```python
from build123d import *

# Parameters (mm, degrees)
EXTRUSION1_DEPTH = 240
ESQUISSE2_R      = 1.5
EXTRUSION2_DEPTH = 242.541404318
ESQUISSE3_W      = 1.5
ESQUISSE3_H      = 20
EXTRUSION3_DEPTH = 20
ESQUISSE5_W      = 1.5
ESQUISSE5_H      = 20
EXTRUSION4_DEPTH = 20
ESQUISSE6_R      = 1.5
EXTRUSION5_DEPTH = 262.423506977


with BuildPart() as part:
    # Esquisse1 → Extrusion1 (new body)
    with BuildSketch(Plane.XY):
        Polygon((0, 0), (20, 0), (20, 1.5), (1.5, 1.5), (1.5, 20), (0, 20), align=None)
    extrude(amount=EXTRUSION1_DEPTH)

    # Esquisse2 → Extrusion2 (cut, through all)
    with BuildSketch(Plane(origin=(0, 1.5, 0), x_dir=(1, 0, 0), z_dir=(0, 1, 0))):
        with Locations(Location((10, -30, 0), (0, 0, 180))):
            Circle(ESQUISSE2_R)
        with Locations(Location((10, -210, 0), (0, 0, 180))):
            Circle(ESQUISSE2_R)
        with Locations(Location((10, -130, 0), (0, 0, 180))):
            Circle(ESQUISSE2_R)
    extrude(amount=-EXTRUSION2_DEPTH, mode=Mode.SUBTRACT)

    # Esquisse3 → Extrusion3 (add)
    with BuildSketch(Plane.XY.offset(240)):
        with Locations((0.75, 10)):
            Rectangle(ESQUISSE3_W, ESQUISSE3_H)
    extrude(amount=EXTRUSION3_DEPTH)

    # Esquisse5 → Extrusion4 (add)
    with BuildSketch(Plane(origin=(0, 0, 0), x_dir=(-1, 0, 0), z_dir=(0, 0, -1))):
        with Locations((-0.75, 10)):
            Rectangle(ESQUISSE5_W, ESQUISSE5_H)
    extrude(amount=EXTRUSION4_DEPTH)

    # Esquisse6 → Extrusion5 (cut, through all)
    with BuildSketch(Plane(origin=(1.5, 0, 0), x_dir=(0, 0, -1), z_dir=(1, 0, 0))):
        with Locations(Location((-248.5, 10, 0), (0, 0, 90))):
            Circle(ESQUISSE6_R)
        with Locations(Location((8.5, 10, 0), (0, 0, 90))):
            Circle(ESQUISSE6_R)
        with Locations(Location((-181, 10, 0), (0, 0, 90))):
            Circle(ESQUISSE6_R)
        with Locations(Location((-59, 10, 0), (0, 0, 90))):
            Circle(ESQUISSE6_R)
    extrude(amount=-EXTRUSION5_DEPTH, mode=Mode.SUBTRACT)


solid = part.part
```
Design review of the part built by this model. Coordinates are the model's own, in mm. A direction names the side the tool comes from. Coordinates: 2 decimals unless noted, no trailing zeros. Loops run counter-clockwise (first coordinate to the right, second up) from the corner with the lowest first, then second, coordinate; pieces in that order, holes last. Notation, with made-up numbers: (4, 66) - (48, 66) arc R4 ccw to (48, 70) - close; hole circle Ø4 at (43, 59.5). An arc over 180 degrees is marked (long way). Use CSV: the item, a comma, the result in double quotes. Start each with the question number.
1) Tool access review of faces 1 (the flat face through (11, 1.5, 118)), 2 (the flat face through (10, 0, 122)): name each direction out of +Z, -Z, +X, -X, +Y, -Y from which nothing blocks a thin tool from reaching the whole face with its end or side.
2) Wall thickness on L1, parallel to Z at x = 10, y = 0.5; L2, parallel to Z at x = 0.55, y = 10; L3, parallel to X at y = 0.4, z = 210: over which ranges is each line inside the solid? List them lowest first. Write a range as from..to.
3) Consider section B-B on z = 191.5. Write out the cut boundary in (x, y).
4) Consider section A-A on y = 4.25. Write out the cut boundary in (x, z).
5) Consider section C-C on x = 4.5. Write out the cut boundary in (y, z), then the cut area to 3 significant figures.
6) For pin 1 Ø4 at (y, z) = (10, -8.5) entering from +X; pin 2 Ø0.8 at (x, y) = (13, 0.5) entering from -Z; pin 3 Ø8 at (x, z) = (11.5, 90.5) entering from +Y; pin 4 Ø2.5 at (x, z) = (10, 30) entering from -Y, all flat-tipped, find the tip position at first contact; note any pin that passes through.
Geometry says:
1,face 1,"+Z, -Z, +X, +Y"
1,face 2,"+Z, -Z, +X, -X, -Y"
2,L1,"0..28.5, 31.5..128.5, 131.5..208.5, 211.5..240"
2,L2,"-20..-10, -7..57.5, 60.5..179.5, 182.5..247, 250..260"
2,L3,"0..8.5, 11.5..20"
3,outline,"(0, 0) - (20, 0) - (20, 1.5) - (1.5, 1.5) - (1.5, 20) - (0, 20) - close"
4,outline,"(0, -20) - (1.5, -20) - (1.5, 260) - (0, 260) - close"
5,outline,"(0, 0) - (1.5, 0) - (1.5, 240) - (0, 240) - close"
5,area,"360 mm^2"
6,pin 1,"x = 1.5"
6,pin 2,"z = 0"
6,pin 3,"y = 1.5"
6,pin 4,"through"
